Could you check a few things on this model? Use its own coordinates, in mm. Give positions to 0.01 mm unless a question says otherwise; leave off trailing zeros. Write each loop counter-clockwise with the first axis right and the second up, starting at its lowest first coordinate (ties: lowest second). Pieces come first, ordered by that corner, then holes. Notation, with made-up numbers: M -1,78.5 L 45,78.5 A22 cw 45,99.5 Z; hole C 11,54 d4. An arc over 180 degrees is marked long. One line per item, written item: value.
```python
from build123d import *
from build123d.topology import SkipClean

# Parameters (mm, degrees)
ESQUISSE1_R               = 1.5
T_LE_DE_BASE_PLI_E1_DEPTH = 1.5
CONG_1_R                  = 2
CONG_2_R                  = 1
ESQUISSE2_W               = 108
ESQUISSE2_H               = 14
PATTE1_DEPTH              = 1.5
CONG_3_R                  = 2
ENL_V_MAT_EXTRU_1_DEPTH   = 1.5
ESQUISSE6_R               = 1.5
ENL_V_MAT_EXTRU_2_DEPTH   = 1.5
ESQUISSE7_R               = 1.6
ENL_V_MAT_EXTRU_3_DEPTH   = 1.5


# Sheet-metal steps are written as plain solids
with BuildPart() as part:
    # Esquisse1 → Tôle de base pliée1 (new body)
    with BuildSketch(Plane(origin=(0, 0, 0), x_dir=(1, 0, 0), z_dir=(0, 1, 0))):
        with BuildLine():
            Line((0, 14.447178434), (0, 11.947178434))
            ThreePointArc((0, 11.947178434), (-2.206641245, 12.610902903), (-3.680981595, 14.381811226))
            ThreePointArc((-3.680981595, 14.381811226), (-37.5, 36.75), (-71.319018405, 14.381811226))
            ThreePointArc((-71.319018405, 14.381811226), (-75, 11.947178434), (-78.680981595, 14.381811226))
            ThreePointArc((-78.680981595, 14.381811226), (-108.32543803, 36.512128565), (-142.200039192, 21.644171779))
            ThreePointArc((-142.200039192, 21.644171779), (-146.671520698, 20.196670583), (-149.432696519, 24))
            Line((-149.432696519, 24), (-149.432696519, 27.828506889))
            ThreePointArc((-149.432696519, 27.828506889), (-151.994672595, 32.376640695), (-154.418263169, 37))
            Line((-154.418263169, 37), (-139, 37))
            Line((-139, 37), (-139, 55))
            Line((-139, 55), (0, 55))
            Line((0, 55), (0, 17.447178434))
            ThreePointArc((0, 17.447178434), (-1.5, 15.947178434), (0, 14.447178434))
        make_face()
        with Locations(Location((-145.432696519, 24, 0), (0, 0, 270))):
            Circle(ESQUISSE1_R, mode=Mode.SUBTRACT)
        with Locations(Location((-75, 15.947178434, 0), (0, 0, 270))):
            Circle(ESQUISSE1_R, mode=Mode.SUBTRACT)
    extrude(amount=-T_LE_DE_BASE_PLI_E1_DEPTH)

    # Congé1
    cong_1_edges = [part.edges().sort_by_distance(p)[0] for p in [
        (-149.432696519, -0.75, -27.828506889),
        (-139, -0.75, -37),
        (-139, -0.75, -55),
    ]]
    fillet(cong_1_edges, radius=CONG_1_R)

    # Congé2
    cong_2_edges = [part.edges().sort_by_distance(p)[0] for p in [
        (-154.418263169, -0.75, -37),
    ]]
    fillet(cong_2_edges, radius=CONG_2_R)

    # Esquisse2 → Patte1 (add)
    with BuildSketch(Plane(origin=(0, 0, 0), x_dir=(1, 0, 0), z_dir=(0, 1, 0))):
        with Locations((-54, 62)):
            Rectangle(ESQUISSE2_W, ESQUISSE2_H)
    extrude(amount=-PATTE1_DEPTH)

    # Congé3
    cong_3_edges = [part.edges().sort_by_distance(p)[0] for p in [
        (-108, -0.75, -55),
        (-108, -0.75, -69),
    ]]
    fillet(cong_3_edges, radius=CONG_3_R)

    # Esquisse5 → Enlèv. mat.-Extru.1 (cut)
    with BuildSketch(Plane(origin=(0, 0, 0), x_dir=(1, 0, 0), z_dir=(0, 1, 0))):
        with BuildLine():
            Line((0, 69), (-52, 69))
            add(Edge.make_bspline(
                [(-52, 69), (-40, 55), (0, 55)],
                knots=[3.446285308, 3.446285308, 3.446285308, 4.71238898, 4.71238898, 4.71238898], degree=2, weights=[1, 0.806225775, 1]))
            Line((0, 55), (0, 69))
        make_face()
    extrude(amount=-ENL_V_MAT_EXTRU_1_DEPTH, mode=Mode.SUBTRACT)

    # Symétrie1: part across face


with BuildPart() as part_1:
    with SkipClean():  # the faces are left unmerged after this step: merging them gives an invalid solid
        add(part.part)
        add(part.part.mirror(Plane(origin=(0, -0.75, -36.223589217), x_dir=(0, 0, 1), z_dir=(1, 0, 0))))

    # Esquisse6 → Enlèv. mat.-Extru.2 (cut)
    with SkipClean():  # the faces are left unmerged after this step: merging them gives an invalid solid
        with BuildSketch(Plane(origin=(0, 0, 0), x_dir=(1, 0, 0), z_dir=(0, 1, 0))):
            with Locations(Location((-84.5, 51.25, 0), (0, 0, 270))):
                Circle(ESQUISSE6_R)
            with Locations(Location((-69.5, 51.25, 0), (0, 0, 270))):
                Circle(ESQUISSE6_R)
            with Locations(Location((84.5, 51.25, 0), (0, 0, 90))):
                Circle(ESQUISSE6_R)
            with Locations(Location((69.5, 51.25, 0), (0, 0, 90))):
                Circle(ESQUISSE6_R)
            with Locations(Location((-130, 51.25, 0), (0, 0, 270))):
                Circle(ESQUISSE6_R)
            with Locations(Location((130, 51.25, 0), (0, 0, 90))):
                Circle(ESQUISSE6_R)
            with Locations(Location((-15, 51.25, 0), (0, 0, 270))):
                Circle(ESQUISSE6_R)
            with Locations(Location((15, 51.25, 0), (0, 0, 90))):
                Circle(ESQUISSE6_R)
        extrude(amount=-ENL_V_MAT_EXTRU_2_DEPTH, mode=Mode.SUBTRACT)

    # Esquisse7 → Enlèv. mat.-Extru.3 (cut)
    with SkipClean():  # the faces are left unmerged after this step: merging them gives an invalid solid
        with BuildSketch(Plane(origin=(0, 0, 0), x_dir=(1, 0, 0), z_dir=(0, 1, 0))):
            with Locations(Location((-89, 62, 0), (0, 0, 270))):
                Circle(ESQUISSE7_R)
            with Locations(Location((-66, 62, 0), (0, 0, 270))):
                Circle(ESQUISSE7_R)
            with Locations(Location((89, 62, 0), (0, 0, 90))):
                Circle(ESQUISSE7_R)
            with Locations(Location((66, 62, 0), (0, 0, 90))):
                Circle(ESQUISSE7_R)
        extrude(amount=-ENL_V_MAT_EXTRU_3_DEPTH, mode=Mode.SUBTRACT)


solid = part_1.part
```
1) Please list where these lines run through material, in increasing order: L1, parallel to Z at x = 89, y = -0.35; L2, parallel to X at y = -0.05, z = -33; L3, parallel to X at y = -1.4, z = -15. Write a range as from..to.
Outcome:
L1: z = -69..-63.6, -60.4..-28.25
L2: x = -152.33..-128.67, -96.33..-53.67, -21.33..21.33, 53.67..96.33, 128.67..152.33
L3: x = -78.95..-76.16, -73.84..-71.05, -3.95..-1.16, 1.16..3.95, 71.05..73.84, 76.16..78.95
2) If we section it at A-A, the plane y = -1.05: Give the number of separate pieces and of enclosed holes in the cut face, then the cut area to 3 significant figures.
Outcome:
separate pieces: 1
enclosed holes: 17
area: 9,250 mm^2
3) I'm going to push flat-ended pins straight in: pin 1 (5 mm diameter, centred on x = -75, z = -15.95, fed in from +Y); pin 2 (0.8 mm diameter, centred on x = -120, y = -0.5, fed in from -Z); pin 3 (0.8 mm diameter, centred on y = -1, z = -25, fed in from -X). Where does each tip first touch, or does it pass through?
Outcome:
pin 1: stops at y = 0
pin 2: stops at z = -55
pin 3: stops at x = -149.43
4) If we section it at B-B, the plane x = -122: Write out the boundary of the cut face in (y, z), then the cut area to 3 significant figures.
Outcome:
outline: M -1.5,-55 L 0,-55 L 0,-35.5 L -1.5,-35.5 Z
area: 29.2 mm^2
5) We'd pull the mould along X, two halves only. Please class faces 1 (the face through (2, 0, -47)), 2 (the face through (-36.899, -0.74, -36.745)): pulls with the +X half, pulls with the -X half, needs draft (parallel to the pull), parting line crosses it, or undercut.
Outcome:
face 1: needs draft
face 2: undercut
